from build123d import *

# Parameters (mm, degrees)
BOSS_EXTRUDE1_DEPTH = 20
CUT_EXTRUDE1_DEPTH  = 88.887054459
CUT_EXTRUDE2_DEPTH  = 102.109516572
LPATTERN1_COUNT     = 6
LPATTERN1_PITCH     = 4.166666667
FILLET1_R           = 0.5
FILLET2_R           = 7.5


with BuildPart() as part:
    # Sketch1 → Boss-Extrude1 (new, symmetric)
    with BuildSketch(Plane(origin=(0, 0, 0), x_dir=(1, 0, 0), z_dir=(0, 1, 0))):
        with BuildLine():
            Line((0, 50.8), (15, 50.8))
            Line((15, 50.8), (15, 25.8))
            Line((15, 25.8), (13, 25.8))
            Line((13, 25.8), (13, 20))
            ThreePointArc((13, 20), (9.464466094, 11.464466094), (18, 15))
            Line((18, 15), (77.733482757, 15))
            Line((77.733482757, 15), (77.733482757, 0))
            Line((77.733482757, 0), (26.228756555, 0))
            ThreePointArc((26.228756555, 0), (-2.099775281, 1.885245467), (0, 30.198684154))
            Line((0, 30.198684154), (0, 50.8))
        make_face()
    extrude(amount=BOSS_EXTRUDE1_DEPTH, both=True)

    # Sketch2 → Cut-Extrude1 (cut, through all)
    with BuildSketch(Plane(origin=(0, 0, -15), x_dir=(-1, 0, 0), z_dir=(0, 0, -1))):
        Polygon((-48.710580838, 0), (-63.173205081, 8.35), (-63.173205081, -8.35), align=None)
    extrude(amount=-CUT_EXTRUDE1_DEPTH, mode=Mode.SUBTRACT)

    # Sketch3 → Cut-Extrude2 (cut, through all)
    with BuildSketch(Plane(origin=(0, 20, 0), x_dir=(1, 0, 0), z_dir=(0, 1, 0))):
        Polygon((15, 25.8), (12.5, 29.966666667), (15, 29.966666667), align=None)
    cut_extrude2 = extrude(amount=-CUT_EXTRUDE2_DEPTH, mode=Mode.SUBTRACT)

    # LPattern1: Cut-Extrude2 ×6
    with Locations(*[(0, 0, -i * LPATTERN1_PITCH) for i in range(1, LPATTERN1_COUNT)]):
        add(cut_extrude2, mode=Mode.SUBTRACT)

    # Fillet1
    fillet1_edges = [part.edges().sort_by_distance(p)[0] for p in [
        (12.5, 0, -46.633333333),
        (13, 0, -25.8),
        (12.5, 0, -29.966666667),
        (12.5, 0, -34.133333333),
        (12.5, 0, -42.466666667),
        (12.5, 0, -38.3),
    ]]
    fillet(fillet1_edges, radius=FILLET1_R)

    # Fillet2
    fillet2_edges = [part.edges().sort_by_distance(p)[0] for p in [
        (12.5, 0, -50.8),
        (77.733482757, 0, -15),
        (77.733482757, 0, 0),
        (26.228756555, 0, 0),
        (0, 0, -30.198684154),
        (0, 0, -50.8),
        (13, 0, -20),
        (18, 0, -15),
    ]]
    fillet(fillet2_edges, radius=FILLET2_R - 0.0001)  # a hair under: the kernel refuses the full size


solid = part.part
Work out the finished part from the listing and answer in its coordinate system (mm). A direction names the side the tool comes from. Give positions to 0.01 mm unless a question says otherwise; leave off trailing zeros. Loops run counter-clockwise (first coordinate to the right, second up) from the corner with the lowest first, then second, coordinate; pieces in that order, holes last. Notation, with made-up numbers: (-33, 52) -> (19, 52) arc R13 cw to (19, 61) -> close; hole circle Ø4 at (44, -10). An arc over 180 degrees is marked (long way). Use a Markdown table: item, result. Add a question column.
1) The part is cut by section D-D, the plane z = -1. Determine the outline of the cut face in (x, y).
2) Consider line 1 along Z through (x, y) = (48.5, -13.5); line 2 along X through (y, z) = (2.5, -12); line 3 along X through (y, z) = (-9, -43). Determine where each line is inside the solid, lowest interval first.
3) For a pull along Z with two mould halves and no side action, classify faces 1 (the cylindrical face through (26.58, 0.28, 0.34)), 2 (the cylindrical face through (12.23, -0.28, -21.69)), 3 (the flat face through (46, 0, -15)), 4 (the flat face through (26, -20, -13)) as +Z half, -Z half, draft (parallel to the pull), parting line (faces both ways), or undercut.
4) Each of these flat-tipped pins is pushed along its axis until it touches: P1, Ø8, axis at y = -7, z = -39.5, coming from the -X side; P2, Ø5, axis at y = -15.5, z = -41, coming from the +X side; P3, Ø0.8, axis at x = 14, y = 1.5, coming from the +Z side; P4, Ø12, axis at x = 57.5, z = -16, coming from the -Y side. Where does it stop, or does it pass through?
5) Which of the six approach directions +Z, -Z, +X, -X, +Y, -Y give full straight-line access (tool end or side, diameter ignored) to faces 5 (the flat face through (45, 0, 0)), 6 (the cylindrical face through (-0.507, 0.28, -30.619)), 7 (the flat face through (13.99, 0.28, -31.65)), 8 (the cylindrical face through (19.602, -0.28, -14.186)), 9 (the flat face through (63.173, 0, -8))?
6) The part is cut by section A-A, the plane z = -14. Determine the outline of the cut face in (x, y).
7) The part is cut by section B-B, the plane x = 58.5. Determine the outline of the cut face in (y, z).
Reported:
| question | item | result |
|---|---|---|
| 1 | outline | (-1.28, -20) -> (73.98, -20) -> (73.98, 20) -> (-1.28, 20) -> close; hole (48.71, 0) -> (63.17, -8.35) -> (63.17, 8.35) -> close |
| 2 | line 1 | z = -15 to 0 |
| 2 | line 2 | x = -6.77 to 9, 17 to 53.04, 63.17 to 76.23 |
| 2 | line 3 | x = 0 to 14.68 |
| 3 | face 1 | +Z half |
| 3 | face 2 | undercut |
| 3 | face 3 | -Z half |
| 3 | face 4 | draft |
| 4 | P1 | stops at x = 0 |
| 4 | P2 | stops at x = 15 |
| 4 | P3 | stops at z = 4.99 |
| 4 | P4 | stops at y = -20 |
| 5 | face 5 | +Z, +X, +Y, -Y |
| 5 | face 6 | -Z, -X, +Y, -Y |
| 5 | face 7 | +X, +Y, -Y |
| 5 | face 8 | -Z, +Y, -Y |
| 5 | face 9 | +Z, -Z |
| 6 | outline | (-6.97, -20) -> (8.1, -20) -> (8.1, 20) -> (-6.97, 20) -> close; (19.26, -20) -> (73.98, -20) -> (73.98, 20) -> (19.26, 20) -> close; hole (48.71, 0) -> (63.17, -8.35) -> (63.17, 8.35) -> close |
| 7 | outline | (-20, -15) -> (-5.65, -15) -> (-5.65, 0) -> (-20, 0) -> close; (5.65, -15) -> (20, -15) -> (20, 0) -> (5.65, 0) -> close |
